Model file for the job. Use its own axes, mm. Give positions to 0.01 mm unless a question says otherwise; leave off trailing zeros. Loops run counter-clockwise (first coordinate to the right, second up) from the corner with the lowest first, then second, coordinate; pieces in that order, holes last. Notation, with made-up numbers: (-13.5, 66) -> (28.5, 66) arc R22 cw to (28.5, 87) -> close; hole circle Ø2 at (68.25, 71.5). An arc over 180 degrees is marked (long way). Use CSV: the item, a comma, the result in double quotes. Start each with the question number.
(1) Cut at D-D on x = 12.5. Write the cut outline in (y, z).
(2) Drill centre lines: probe 1 along Y at (x, z) = (6.25, 0.3); probe 2 along X at (y, z) = (1, 0.95); probe 3 along Y at (x, z) = (0, 0.45). Where is each one in solid material? Low to high.
(3) Cut at C-C on z = 0.7. State how many separate pieces and enclosed holes the cut face has, then the cut area to 3 significant figures.
(4) Cut at A-A on y = 0. Write the cut outline in (x, z), then the cut area to 3 significant figures.
(5) Flat gauge pin, fed straight in: pin 1 (3 mm diameter, centred on x = 8.83, y = -5.1, fed in from -Z). Where does the tip first touch, or does it go through?
(6) Cut at B-B on x = 0. Write the cut outline in (y, z).
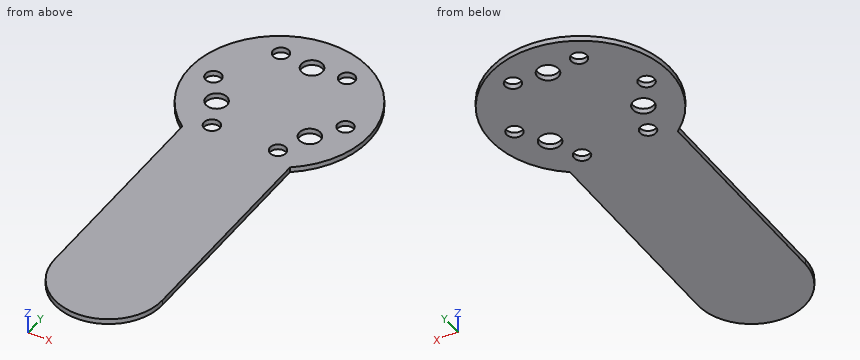
from build123d import *

# Parameters (mm, degrees)
SKETCH2_R           = 2
SKETCH2_R_2         = 1.5
BOSS_EXTRUDE2_DEPTH = 1


with BuildPart() as part:
    # Sketch2 → Boss-Extrude2 (new body)
    with BuildSketch(Plane.XY):
        with BuildLine():
            Line((-10.2, -13.6), (-10.2, -53.6))
            ThreePointArc((-10.2, -53.6), (0, -63.8), (10.2, -53.6))
            Line((10.2, -53.6), (10.2, -13.6))
            ThreePointArc((10.2, -13.6), (0, 17), (-10.2, -13.6))
        make_face()
        with Locations((0, 10.2)):
            Circle(SKETCH2_R, mode=Mode.SUBTRACT)
        with Locations((8.833459119, -5.1)):
            Circle(SKETCH2_R, mode=Mode.SUBTRACT)
        with Locations((-8.833459119, -5.1)):
            Circle(SKETCH2_R, mode=Mode.SUBTRACT)
        with Locations((-12.5, 0)):
            Circle(SKETCH2_R_2, mode=Mode.SUBTRACT)
        with Locations((-6.25, 10.825317547)):
            Circle(SKETCH2_R_2, mode=Mode.SUBTRACT)
        with Locations((6.25, 10.825317547)):
            Circle(SKETCH2_R_2, mode=Mode.SUBTRACT)
        with Locations((12.5, 0)):
            Circle(SKETCH2_R_2, mode=Mode.SUBTRACT)
        with Locations((6.25, -10.825317547)):
            Circle(SKETCH2_R_2, mode=Mode.SUBTRACT)
        with Locations((-6.25, -10.825317547)):
            Circle(SKETCH2_R_2, mode=Mode.SUBTRACT)
    extrude(amount=BOSS_EXTRUDE2_DEPTH)


solid = part.part
Check result:
1,outline,"(-11.52, 0) -> (-1.5, 0) -> (-1.5, 1) -> (-11.52, 1) -> close; (1.5, 0) -> (11.52, 0) -> (11.52, 1) -> (1.5, 1) -> close"
2,probe 1,"-61.66 to -12.33, -9.33 to 9.33, 12.33 to 15.81"
2,probe 2,"-16.97 to -13.62, -11.38 to 11.38, 13.62 to 16.97"
2,probe 3,"-63.8 to 8.2, 12.2 to 17"
3,separate pieces,"1"
3,enclosed holes,"9"
3,area,"1,760 mm²"
4,outline,"(-17, 0) -> (-14, 0) -> (-14, 1) -> (-17, 1) -> close; (-11, 0) -> (11, 0) -> (11, 1) -> (-11, 1) -> close; (14, 0) -> (17, 0) -> (17, 1) -> (14, 1) -> close"
4,area,"28.0 mm²"
5,pin 1,"through"
6,outline,"(-63.8, 0) -> (8.2, 0) -> (8.2, 1) -> (-63.8, 1) -> close; (12.2, 0) -> (17, 0) -> (17, 1) -> (12.2, 1) -> close"
